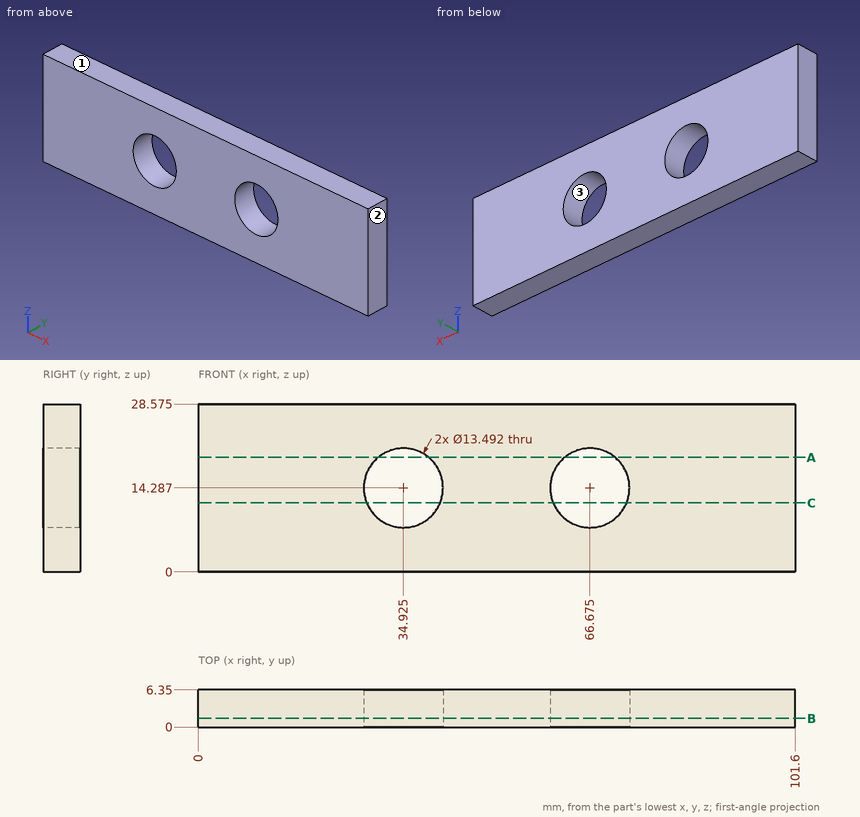
Geometry: see drawing. Coordinates: mm, zero at the bounding-box minimum. Give positions to 0.01 mm unless a question says otherwise; leave off trailing zeros. Order: outer loops, then holes, each group sorted by start corner. A loop starts at its lowest first (then second) coordinate and runs counter-clockwise, first axis right, second up. Notation, with made-up numbers: (0, 2) - (39, 2) arc R18 ccw to (39, 17) - close; hole circle Ø8 at (49.25, 2.25). An arc over 180 degrees is marked (long way). Use CSV: the item, a comma, the result in double quotes.
1. Mould query, pull axis Z, two halves, no side actions, for the marked faces 1, 2 and 3. Classes: +Z half, -Z half, draft (parallel to the pull), parting line (faces both ways), or undercut.
Answers below:
face 1,"+Z half"
face 2,"draft"
face 3,"undercut"
2. Section query C-C (z = 11.75). Give the number of separate pieces and of enclosed holes in the cut face.
Answers below:
separate pieces,"3"
enclosed holes,"0"
3. Section query B-B (y = 1.5). Output: boundary loops of the cut face in (x, z) (1 decimal), plus the area to 3 significant figures.
Answers below:
outline,"(0, 0) - (101.6, 0) - (101.6, 28.6) - (0, 28.6) - close; hole circle Ø13.5 at (34.9, 14.3); hole circle Ø13.5 at (66.7, 14.3)"
area,"2,620 mm2"
4. Section query A-A (z = 19.5). Output: boundary loops of the cut face in (x, y).
Answers below:
outline,"(0, 0) - (30.64, 0) - (30.64, 6.35) - (0, 6.35) - close; (39.21, 0) - (62.39, 0) - (62.39, 6.35) - (39.21, 6.35) - close; (70.96, 0) - (101.6, 0) - (101.6, 6.35) - (70.96, 6.35) - close"
5. Material intervals for line 1 along X through (y, z) = (5.5, 14) (1 decimal); line 2 along X through (y, z) = (1, 16.5); line 3 along Z through (x, y) = (36, 2) (1 decimal), sorted ascending. Write a range as from..to.
Answers below:
line 1,"0..28.2, 41.7..59.9, 73.4..101.6"
line 2,"0..28.55, 41.3..60.3, 73.05..101.6"
line 3,"0..7.6, 20.9..28.6"
